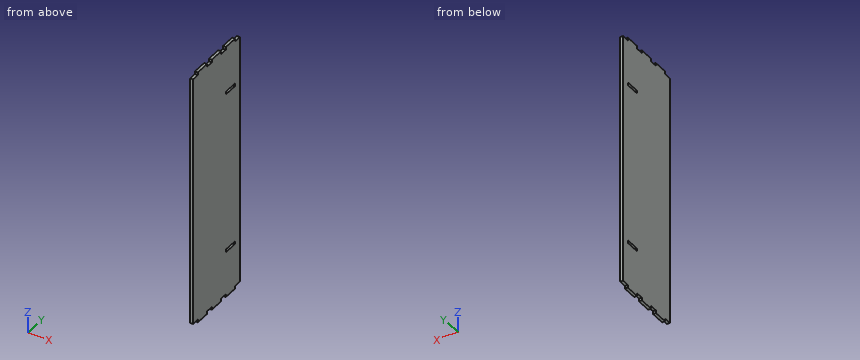
from build123d import *

# Parameters (mm, degrees)
SKETCH1_W               = 279.4
SKETCH1_H               = 76.2
BOSS_EXTRUDE1_DEPTH     = 3
SKETCH3_W               = 3
SKETCH3_H               = 7.8
CUT_EXTRUDE1_DEPTH      = 145.833352512
LPATTERN1_COUNT         = 4
LPATTERN1_PITCH         = 22.8
MIRROR1_COPY_1_SKETCH_W = 3
MIRROR1_COPY_1_SKETCH_H = 7.8
MIRROR1_COPY_1_DEPTH    = 145.833352512
MIRROR1_COPY_2_SKETCH_W = 3
MIRROR1_COPY_2_SKETCH_H = 7.8
MIRROR1_COPY_2_DEPTH    = 145.833352512
MIRROR1_COPY_3_SKETCH_W = 3
MIRROR1_COPY_3_SKETCH_H = 7.8
MIRROR1_COPY_3_DEPTH    = 145.833352512
SKETCH5_W               = 3
SKETCH5_H               = 15
CUT_EXTRUDE3_DEPTH      = 10


with BuildPart() as part:
    # Sketch1 → Boss-Extrude1 (new body)
    with BuildSketch(Plane(origin=(0, 0, 0), x_dir=(0, 0, -1), z_dir=(1, 0, 0))):
        Rectangle(SKETCH1_W, SKETCH1_H)
    extrude(amount=-BOSS_EXTRUDE1_DEPTH)

    # Sketch3 → Cut-Extrude1 (cut, through all)
    with BuildSketch(Plane.ZY.offset(3)):
        with Locations((-138.2, 34.2)):
            Rectangle(SKETCH3_W, SKETCH3_H)
    cut_extrude1 = extrude(amount=-CUT_EXTRUDE1_DEPTH, mode=Mode.SUBTRACT)

    # LPattern1: Cut-Extrude1 ×4
    with Locations(*[(0, -i * LPATTERN1_PITCH, 0) for i in range(1, LPATTERN1_COUNT)]):
        add(cut_extrude1, mode=Mode.SUBTRACT)

    # Mirror1: Cut-Extrude1 across plane
    add(cut_extrude1.mirror(Plane.XY), mode=Mode.SUBTRACT)

    # Mirror1 copy 1 sketch → Mirror1 copy 1 (cut, through all)
    with BuildSketch(Plane(origin=(-3, -22.8, 0), x_dir=(0, 0, -1), z_dir=(-1, 0, 0))):
        with Locations((-138.2, -34.2)):
            Rectangle(MIRROR1_COPY_1_SKETCH_W, MIRROR1_COPY_1_SKETCH_H)
    extrude(amount=-MIRROR1_COPY_1_DEPTH, mode=Mode.SUBTRACT)

    # Mirror1 copy 2 sketch → Mirror1 copy 2 (cut, through all)
    with BuildSketch(Plane(origin=(-3, -45.6, 0), x_dir=(0, 0, -1), z_dir=(-1, 0, 0))):
        with Locations((-138.2, -34.2)):
            Rectangle(MIRROR1_COPY_2_SKETCH_W, MIRROR1_COPY_2_SKETCH_H)
    extrude(amount=-MIRROR1_COPY_2_DEPTH, mode=Mode.SUBTRACT)

    # Mirror1 copy 3 sketch → Mirror1 copy 3 (cut, through all)
    with BuildSketch(Plane(origin=(-3, -68.4, 0), x_dir=(0, 0, -1), z_dir=(-1, 0, 0))):
        with Locations((-138.2, -34.2)):
            Rectangle(MIRROR1_COPY_3_SKETCH_W, MIRROR1_COPY_3_SKETCH_H)
    extrude(amount=-MIRROR1_COPY_3_DEPTH, mode=Mode.SUBTRACT)

    # Sketch5 → Cut-Extrude3 (cut)
    with BuildSketch(Plane.ZY.offset(3)):
        with Locations((-88.2, 22.8)):
            Rectangle(SKETCH5_W, SKETCH5_H)
    cut_extrude3 = extrude(amount=-CUT_EXTRUDE3_DEPTH, mode=Mode.SUBTRACT)

    # Mirror2: Cut-Extrude3 across plane
    add(cut_extrude3.mirror(Plane.XY), mode=Mode.SUBTRACT)


solid = part.part
Can you work these out from the model? Positions are in its coordinate system, mm. Coordinates: 2 decimals unless noted, no trailing zeros. Write each loop counter-clockwise with the first axis right and the second up, starting at its lowest first coordinate (ties: lowest second). Pieces come first, ordered by that corner, then holes. Notation, with made-up numbers: (43, -5.75) -> (81, -5.75) arc R18 cw to (81, 29.25) -> close; hole circle Ø7 at (-26, 10.25). An arc over 180 degrees is marked (long way). Write item = value, one per line.
(1) If I drill on probe 1 along Z at (x, y) = (-2.9, 16); probe 2 along Z at (x, y) = (-1.15, -34), over which ranges is the centre line in solid material (lowest first)?
Verdict:
probe_1 = -139.7 to -89.7, -86.7 to 86.7, 89.7 to 139.7
probe_2 = -136.7 to 136.7
(2) For pin 1 (1.5 mm diameter, centred on x = -1.5, y = 10, fed in from -Z); pin 2 (2 mm diameter, centred on y = 23, z = 35, fed in from +X); pin 3 (1.5 mm diameter, centred on x = -1.5, z = -137.5, fed in from +Y); pin 4 (1.5 mm diameter, centred on x = -1.5, z = 137.5, fed in from -Y), each with a flat end and sliding along its axis, tell me the tip position at first contact or that it passes through.
Verdict:
pin_1 = -136.7
pin_2 = 0
pin_3 = 30.3
pin_4 = -30.3
(3) Imagine slicing it at A-A (y = -10). Please give me the cut outline in (x, z).
Verdict:
outline = (-3, -136.7) -> (0, -136.7) -> (0, 136.7) -> (-3, 136.7) -> close
